The model under review builds one solid part; all positions refer to its coordinate system, in mm. Face numbers are marked on the shaded views. A direction names the side the tool comes from. Coordinates: 2 decimals unless noted, no trailing zeros. Order: outer loops, then holes, each group sorted by start corner. A loop starts at its lowest first (then second) coordinate and runs counter-clockwise, first axis right, second up. Notation, with made-up numbers: (36, 59) -> (79, 59) arc R15 cw to (79, 68) -> close; hole circle Ø2 at (-38.5, 39.25). An arc over 180 degrees is marked (long way). Use one line per item in the form item = value. Start each with the question number.
(1) Take a section at B-B (y = 8). State the section outline as (x, z) points.
(2) Take a section at D-D (x = -22.5). State the section outline as (y, z) points.
(3) For the marked faces 1, 2 and 3, list the 3-axis set-ups (+Z, -Z, +X, -X, +Y, -Y) from which the entire face can be reached by the end or side of a thin tool; tool diameter is ignored.
(4) Take a section at A-A (y = 1.9). State the section outline as (x, z) points, then the cut area to 3 significant figures.
(5) Take a section at C-C (z = 13). State the section outline as (x, y) points.
(6) Mouldability with a two-part tool opening along Z and no side actions: class the marked faces 4, 5 and 6 as +Z half, -Z half, draft (parallel to the pull), parting line (faces both ways), or undercut.
(7) Wall thickness on line 1 along Y through (x, z) = (-22.5, 3.55); line 2 along Y through (x, z) = (-35.45, 6.8); line 3 along Y through (x, z) = (-18.75, 2.5): over which ranges is each line inside the solid? List them lowest first.
(8) Insertion check: pin 1 Ø6.5 at (y, z) = (13.2, 19) entering from -X; pin 2 Ø3 at (x, y) = (-29.5, 8) entering from -Z; pin 3 Ø2 at (x, y) = (-22.5, -7) entering from -Z; pin 4 Ø2 at (x, z) = (-26, 4) entering from +Y. Each pin has a flat end and moves straight along its axis. Give the tip position at first contact, or say it passes through.
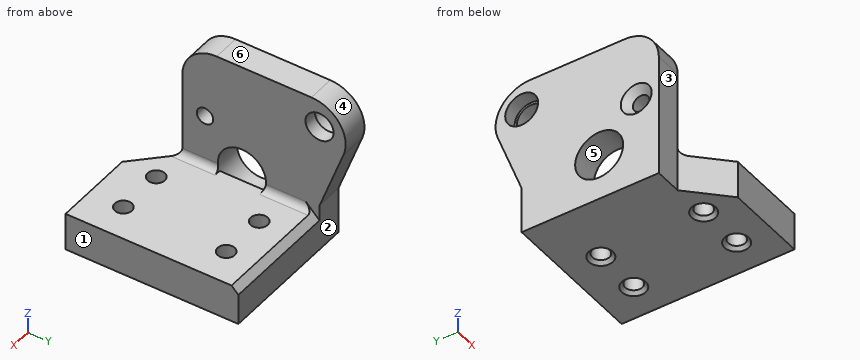
```python
from build123d import *

# Parameters (mm, degrees)
SKETCH_1_W             = 69.5
SKETCH_1_H             = 24
EXTRUDE_1_DEPTH        = 10.5
SKETCH_2_W             = 35
SKETCH_2_H             = 3
CUT_EXTRUDE_2_DEPTH    = 24
HOLE_WIZARD_M3_1_D     = 2.5
HOLE_WIZARD_M3_1_DEPTH = 7.5
HOLE_WIZARD_M3_1_TIP   = 0.751075774
CHAMFER_1_SIZE         = 0.5
CHAMFER_2_SIZE         = 0.5
CHAMFER_3_SIZE         = 5.2
FILLET1_R              = 2
SKETCH_8_W             = 10.5
SKETCH_8_H             = 1.2
EXTRUDE_1_2_DEPTH      = 69.5
SKETCH_7_W             = 35
SKETCH_7_H             = 30
CUT_EXTRUDE_1_DEPTH    = 71.5
FILLET_1_R             = 2
FILLET_2_R             = 2
SKETCH2_W              = 16.266114445
SKETCH2_H              = 35.800653755
SKETCH2_W_2            = 16.722173729
SKETCH2_H_2            = 38.308979815
EXTRUDE1_DEPTH         = 5
SKETCH4_R              = 2.05
SKETCH4_R_2            = 3.5
EXTRUDE2_DEPTH         = 4
FILLET2_R              = 5
SKETCH7_R              = 3.5
SKETCH7_R_2            = 2.05
EXTRUDE3_DEPTH         = 4
FILLET3_R              = 5
FILLET5_R              = 1
SKETCH14_R             = 2.4
EXTRUDE4_DEPTH         = 2
SKETCH15_R             = 2.4
EXTRUDE5_DEPTH         = 2
SKETCH_9_W             = 36.650882696
SKETCH_9_H             = 47.613245362
CUT_EXTRUDE_2_2_DEPTH  = 49.168282868
SKETCH_10_W            = 16.727542875
SKETCH_10_H            = 39.365484233
CUT_EXTRUDE_3_DEPTH    = 5
CHAMFER_8_SIZE         = 1
FILLET_4_R             = 1


with BuildPart() as part:
    # 草图1 → Extrude 1 (new body)
    with BuildSketch(Plane.XY):
        Rectangle(SKETCH_1_W, SKETCH_1_H)
    extrude(amount=EXTRUDE_1_DEPTH)

    # 草图2 → Cut-Extrude 2 (cut)
    with BuildSketch(Plane.XZ.offset(12)):
        with Locations((0, 1.5)):
            Rectangle(SKETCH_2_W, SKETCH_2_H)
    extrude(amount=-CUT_EXTRUDE_2_DEPTH, mode=Mode.SUBTRACT)

    # M3 螺纹孔1
    with Locations(Plane(origin=(22.5, 8, 0), x_dir=(-1, 0, 0), z_dir=(0, 0, -1))):
        with Locations((0, 0), (0, -15), (45, -15), (45, 0), (-7, 0), (-7, -15), (52, -15), (52, 0)):
            Hole(HOLE_WIZARD_M3_1_D / 2, depth=HOLE_WIZARD_M3_1_DEPTH)
            with Locations((0, 0, -(HOLE_WIZARD_M3_1_DEPTH + HOLE_WIZARD_M3_1_TIP / 2))):  # 118° drill point
                Cone(0, HOLE_WIZARD_M3_1_D / 2, HOLE_WIZARD_M3_1_TIP, mode=Mode.SUBTRACT)

    # 倒角1
    chamfer_1_edges = [part.edges().sort_by_distance(p)[0] for p in [
        (-23.75, 8, 0),
        (-23.75, -7, 0),
        (21.25, -7, 0),
        (21.25, 8, 0),
    ]]
    chamfer(chamfer_1_edges, length=CHAMFER_1_SIZE)

    # 倒角2
    chamfer_2_edges = [part.edges().sort_by_distance(p)[0] for p in [
        (-30.75, 8, 0),
        (-30.75, -7, 0),
        (28.25, -7, 0),
        (28.25, 8, 0),
    ]]
    chamfer(chamfer_2_edges, length=CHAMFER_2_SIZE)

    # 倒角3
    chamfer_3_edges = [part.edges().sort_by_distance(p)[0] for p in [
        (34.75, -12, 5.25),
        (-34.75, -12, 5.25),
    ]]
    chamfer(chamfer_3_edges, length=CHAMFER_3_SIZE)

    # Fillet1
    fillet1_edges = [part.edges().sort_by_distance(p)[0] for p in [
        (0, -12, 10.5),
    ]]
    fillet(fillet1_edges, radius=FILLET1_R)

    # 草图8 → Extrude 1 2 (add)
    with BuildSketch(Plane(origin=(34.75, 0, 0), x_dir=(0, 0, -1), z_dir=(1, 0, 0))):
        with Locations((-5.25, 12.6)):
            Rectangle(SKETCH_8_W, SKETCH_8_H)
    extrude(amount=-EXTRUDE_1_2_DEPTH)

    # 草图7 → 切除-拉伸1 (cut)
    with BuildSketch(Plane.XY.offset(10.5)):
        with Locations((0, 3)):
            Rectangle(SKETCH_7_W, SKETCH_7_H)
    extrude(amount=-CUT_EXTRUDE_1_DEPTH, mode=Mode.SUBTRACT)


with BuildPart() as cut_extrude_1_piece_1:
    # of the separate pieces the step leaves, piece 1, a body of its own (cut_extrude_1_pieces)
    add(part.part.solids().sort_by_distance((29.55, -12, 8.5))[0])

    # 圆角1
    fillet_1_edges = [cut_extrude_1_piece_1.edges().sort_by_distance(p)[0] for p in [
        (26.125, 13.2, 10.5),
    ]]
    fillet(fillet_1_edges, radius=FILLET_1_R)


with BuildPart() as cut_extrude_1_piece_2:
    # of the separate pieces the step leaves, piece 2, a body of its own (cut_extrude_1_pieces)
    add(part.part.solids().sort_by_distance((-29.55, -12, 8.5))[0])

    # 圆角2
    fillet_2_edges = [cut_extrude_1_piece_2.edges().sort_by_distance(p)[0] for p in [
        (-26.125, 13.2, 10.5),
    ]]
    fillet(fillet_2_edges, radius=FILLET_2_R)


with BuildPart() as extrude1_tool:
    # Sketch2 → Extrude1 (new body)
    with BuildSketch(Plane.XY.offset(10.5)):
        with Locations((34.133057222, -0.236108687)):
            Rectangle(SKETCH2_W, SKETCH2_H)
        with Locations((-34.361086865, 1.85416303)):
            Rectangle(SKETCH2_W_2, SKETCH2_H_2)
    extrude(amount=-EXTRUDE1_DEPTH)


with BuildPart() as cut_extrude_1_piece_1_1:
    add(cut_extrude_1_piece_1.part)

    # Extrude1: cut by extrude1_tool
    add(extrude1_tool.part, mode=Mode.SUBTRACT)

    # Sketch7 → Extrude3 (add)
    with BuildSketch(Plane(origin=(34.75, 0, 0), x_dir=(0, 0, -1), z_dir=(1, 0, 0))):
        Polygon((0, -6.797975685), (0, 13.202024315), (-6.8, 13.202024315), (-23, 19.202024315), (-23, -6.797975685), align=None)
        with Locations(Location((-6.8, 1.9, 0), (0, 0, 68.196252011))):
            Circle(SKETCH7_R, mode=Mode.SUBTRACT)
        with Locations(Location((-19, 13.2, 0), (0, 0, 180))):
            Circle(SKETCH7_R_2, mode=Mode.SUBTRACT)
    extrude(amount=EXTRUDE3_DEPTH)

    # Fillet3
    fillet3_edges = [cut_extrude_1_piece_1_1.edges().sort_by_distance(p)[0] for p in [
        (36.75, -6.797975685, 23),
        (36.75, 19.202024315, 23),
    ]]
    fillet(fillet3_edges, radius=FILLET3_R)

    # Sketch12 → CSK for M2 Slotted raised CTSK head wood (revolve, cut)
    with BuildSketch(Plane(origin=(38.75, -3.5, 13), x_dir=(0, 0, -1), z_dir=(0, 1, 0))):
        Polygon((0, 0), (0, 77.5), (1.2, 77.5), (1.2, 1.05), (2.25, 0), align=None)
    revolve(axis=Axis((45.1, -3.5, 13), (-1, 0, 0)), mode=Mode.SUBTRACT)

    # Fillet5
    # the kernel refuses this fillet: 1 mm, written as the material it adds along each edge
    with BuildSketch(Plane(origin=(26, -12, 5.5), x_dir=(1, 0, 0), z_dir=(0, 1, 0))) as fillet5_piece_1:
        with BuildLine():
            CenterArc((FILLET5_R, -FILLET5_R), FILLET5_R, 90, 90)
            Line((0, -FILLET5_R), (0, 0))
            Line((0, 0), (FILLET5_R, 0))
        make_face()
    extrude(amount=25.2)
    with BuildSketch(Plane(origin=(34.75, -6.797975685, 5.5), x_dir=(0, 0, 1), z_dir=(0, 1, 0))) as fillet5_piece_2_section:
        with BuildLine():
            CenterArc((FILLET5_R, -FILLET5_R), FILLET5_R, 90, 90)
            Line((0, -FILLET5_R), (0, 0))
            Line((0, 0), (FILLET5_R, 0))
        make_face()
    fillet5_piece_2 = extrude(amount=7.948360323, mode=Mode.PRIVATE)
    fillet5_piece_2 = fillet5_piece_2 - Plane(origin=(34.525455487, 1.9, 6.8), x_dir=(0, 0.9284615319608756, -0.371428571422372), z_dir=(-1, 0, 0)) * Cylinder(3.5, 20, mode=Mode.PRIVATE)
    add(fillet5_piece_2)
    with BuildSketch(Plane(origin=(34.75, 2.649615362, 5.5), x_dir=(0, 0, 1), z_dir=(0, 1, 0))) as fillet5_piece_3_section:
        with BuildLine():
            CenterArc((FILLET5_R, -FILLET5_R), FILLET5_R, 90, 90)
            Line((0, -FILLET5_R), (0, 0))
            Line((0, 0), (FILLET5_R, 0))
        make_face()
    fillet5_piece_3 = extrude(amount=10.550384638, mode=Mode.PRIVATE)
    fillet5_piece_3 = fillet5_piece_3 - Plane(origin=(34.525839379, 1.9, 6.8), x_dir=(0, 0.9284615319608756, -0.371428571422372), z_dir=(-1, 0, 0)) * Cylinder(3.5, 26, mode=Mode.PRIVATE)
    add(fillet5_piece_3)

    # Sketch15 → Extrude5 (cut)
    with BuildSketch(Plane(origin=(38.75, 0, 0), x_dir=(0, 0, -1), z_dir=(1, 0, 0))):
        with Locations(Location((-19, 13.2, 0), (0, 0, 180))):
            Circle(SKETCH15_R)
    extrude(amount=-EXTRUDE5_DEPTH, mode=Mode.SUBTRACT)

    # 草图9 → Cut-Extrude 2 2 (cut, through all)
    with BuildSketch(Plane.XY.offset(23)):
        with Locations((21.816576683, -0.846593787)):
            Rectangle(SKETCH_9_W, SKETCH_9_H)
    extrude(amount=-CUT_EXTRUDE_2_2_DEPTH, mode=Mode.SUBTRACT)


with BuildPart() as cut_extrude_1_piece_2_1:
    add(cut_extrude_1_piece_2.part)

    # Extrude1: cut by extrude1_tool
    add(extrude1_tool.part, mode=Mode.SUBTRACT)

    # Sketch4 → Extrude2 (add)
    with BuildSketch(Plane.ZY.offset(34.75)):
        Polygon((0, -6.8), (0, 13.2), (6.8, 13.2), (23, 19.2), (23, -6.8), align=None)
        with Locations((19, 13.2)):
            Circle(SKETCH4_R, mode=Mode.SUBTRACT)
        with Locations(Location((6.8, 1.9, 0), (0, 0, 111.803747989))):
            Circle(SKETCH4_R_2, mode=Mode.SUBTRACT)
    extrude(amount=EXTRUDE2_DEPTH)

    # Fillet2
    fillet2_edges = [cut_extrude_1_piece_2_1.edges().sort_by_distance(p)[0] for p in [
        (-36.75, -6.8, 23),
        (-36.75, 19.2, 23),
    ]]
    fillet(fillet2_edges, radius=FILLET2_R)

    # Sketch13 → CSK for M2 Slotted raised CTSK head  2 (revolve, cut)
    with BuildSketch(Plane(origin=(-38.75, -3.5, 13), x_dir=(0, 0, 1), z_dir=(0, 1, 0))):
        Polygon((0, 0), (0, 4), (1.2, 4), (1.2, 1.05), (2.25, 0), align=None)
    revolve(axis=Axis((-45.1, -3.5, 13), (1, 0, 0)), mode=Mode.SUBTRACT)

    # Sketch14 → Extrude4 (cut)
    with BuildSketch(Plane.ZY.offset(38.75)):
        with Locations((19, 13.2)):
            Circle(SKETCH14_R)
    extrude(amount=-EXTRUDE4_DEPTH, mode=Mode.SUBTRACT)

    # 草图10 → 切除-拉伸3 (cut)
    with BuildSketch(Plane.XY.offset(10.5)):
        with Locations((-20.237373351, 1.950530044)):
            Rectangle(SKETCH_10_W, SKETCH_10_H)
    extrude(amount=-CUT_EXTRUDE_3_DEPTH, mode=Mode.SUBTRACT)

    # 倒角8
    chamfer_8_edges = [cut_extrude_1_piece_2_1.edges().sort_by_distance(p)[0] for p in [
        (-26.125, 13.2, 5.5),
    ]]
    chamfer(chamfer_8_edges, length=CHAMFER_8_SIZE)

    # 圆角4
    # the kernel refuses this fillet: 1 mm, written as the material it adds along each edge
    with BuildSketch(Plane(origin=(-34.75, 14.7, 5.5), x_dir=(0, 0, 1), z_dir=(0, -1, 0))) as fillet_4_piece_1_section:
        with BuildLine():
            CenterArc((FILLET_4_R, -FILLET_4_R), FILLET_4_R, 90, 90)
            Line((0, -FILLET_4_R), (0, 0))
            Line((0, 0), (FILLET_4_R, 0))
        make_face()
    fillet_4_piece_1 = extrude(amount=12.050384638, mode=Mode.PRIVATE)
    fillet_4_piece_1 = fillet_4_piece_1 - Plane(origin=(-34.522632455, 1.9, 6.8), x_dir=(0, 0.9284615319608756, -0.3714285714223719), z_dir=(1, 0, 0)) * Cylinder(3.5, 29, mode=Mode.PRIVATE)
    fillet_4_piece_1 = split(fillet_4_piece_1, bisect_by=Plane(origin=(-34.522632455, 10.293168588, 7.406831412), z_dir=(0, -0.7071067811865476, -0.7071067811865476)), keep=Keep.TOP, mode=Mode.PRIVATE)
    add(fillet_4_piece_1)
    with BuildSketch(Plane(origin=(-34.75, 1.150384638, 5.5), x_dir=(0, 0, 1), z_dir=(0, -1, 0))) as fillet_4_piece_2_section:
        with BuildLine():
            CenterArc((FILLET_4_R, -FILLET_4_R), FILLET_4_R, 90, 90)
            Line((0, -FILLET_4_R), (0, 0))
            Line((0, 0), (FILLET_4_R, 0))
        make_face()
    fillet_4_piece_2 = extrude(amount=10.450384638, mode=Mode.PRIVATE)
    fillet_4_piece_2 = split(fillet_4_piece_2, bisect_by=Plane(origin=(-35.981733075, -5.568266925, 5.72144918), z_dir=(0.7071067811865476, 0.7071067811865475, 0)), keep=Keep.TOP, mode=Mode.PRIVATE)
    fillet_4_piece_2 = fillet_4_piece_2 - Plane(origin=(-34.525455927, 1.9, 6.8), x_dir=(0, 0.9284615319608756, -0.3714285714223719), z_dir=(1, 0, 0)) * Cylinder(3.5, 25, mode=Mode.PRIVATE)
    add(fillet_4_piece_2)


solid = cut_extrude_1_piece_2_1.part
```
Findings:
q1.outline = (-38.75, 0) -> (-31.25, 0) -> (-30.75, 0.5) -> (-30.75, 5.5) -> (-33.75, 5.5) arc R1 cw to (-34.75, 6.5) -> (-34.75, 23) -> (-38.75, 23) -> close; (-28.25, 0.5) -> (-27.75, 0) -> (-24.25, 0) -> (-23.75, 0.5) -> (-23.75, 5.5) -> (-28.25, 5.5) -> close; (-21.25, 0.5) -> (-20.75, 0) -> (-17.5, 0) -> (-17.5, 5.5) -> (-21.25, 5.5) -> close
q2.outline = (-12, 0) -> (-8.75, 0) -> (-8.25, 0.5) -> (-8.25, 5.5) -> (-12, 5.5) -> close; (-5.75, 0.5) -> (-5.25, 0) -> (6.25, 0) -> (6.75, 0.5) -> (6.75, 5.5) -> (-5.75, 5.5) -> close; (9.25, 0.5) -> (9.75, 0) -> (13.2, 0) -> (13.2, 4.5) -> (12.2, 5.5) -> (9.25, 5.5) -> close
q3.face_1 = +Z, -Z, +X, +Y, -Y
q3.face_2 = -Z, +X, -X, +Y
q3.face_3 = +Z, -Z, -X, -Y
q4.outline = (-38.75, 0) -> (-17.5, 0) -> (-17.5, 5.5) -> (-34.75, 5.5) -> (-34.75, 3.3) -> (-38.75, 3.3) -> close; (-38.75, 10.3) -> (-34.75, 10.3) -> (-34.75, 23) -> (-38.75, 23) -> close
q4.area = 159 mm²
q5.outline = (-38.75, -6.8) -> (-34.75, -6.8) -> (-34.75, -4.7) -> (-37.7, -4.7) -> (-38.75, -5.75) -> close; (-38.75, -1.25) -> (-37.7, -2.3) -> (-34.75, -2.3) -> (-34.75, 15.5) -> (-38.75, 15.5) -> close
q6.face_4 = parting line
q6.face_5 = undercut
q6.face_6 = +Z half
q7.line_1 = -12 to -8.25, -5.75 to 6.75, 9.25 to 13.2
q7.line_2 = -6.8 to -1.6, 5.4 to 13.2
q7.line_3 = -12 to 13.2
q8.pin_1 = -38.75
q8.pin_2 = 0.25
q8.pin_3 = through
q8.pin_4 = 13.2
